The listing builds one solid part. Answer for the finished solid, in the listing's coordinates (mm). A direction names the side the tool comes from. Coordinates: 2 decimals unless noted, no trailing zeros. Loops run counter-clockwise (first coordinate to the right, second up) from the corner with the lowest first, then second, coordinate; pieces in that order, holes last. Notation, with made-up numbers: (15, 15) -> (38, 15) arc R32 cw to (38, 50) -> close; hole circle Ø4 at (18.25, 68). An arc over 180 degrees is marked (long way). Answer in a Markdown table with one row per item.
```python
from build123d import *

# Parameters (mm, degrees)
SKETCH1_R           = 50.8
SKETCH1_R_2         = 12.7
BOSS_EXTRUDE1_DEPTH = 3


with BuildPart() as part:
    # Sketch1 → Boss-Extrude1 (new body)
    with BuildSketch(Plane(origin=(0, 0, 0), x_dir=(1, 0, 0), z_dir=(0, 1, 0))):
        Circle(SKETCH1_R)
        Circle(SKETCH1_R_2, mode=Mode.SUBTRACT)
        with BuildLine():
            ThreePointArc((-33.25, 0), (-23.511300474, -23.511300474), (0, -33.25))
            ThreePointArc((0, -33.25), (1.5, -31.75), (0, -30.25))
            ThreePointArc((0, -30.25), (-21.389980131, -21.389980131), (-30.25, 0))
            ThreePointArc((-30.25, 0), (-31.75, 1.5), (-33.25, 0))
        make_face(mode=Mode.SUBTRACT)
        with BuildLine():
            ThreePointArc((-26.373662173, 5.295275591), (-19.021172414, -19.021172414), (5.295275591, -26.373662173))
            ThreePointArc((5.295275591, -26.373662173), (6.470650307, -24.607736275), (4.704724409, -23.432361559))
            ThreePointArc((4.704724409, -23.432361559), (-16.89985207, -16.89985207), (-23.432361559, 4.704724409))
            ThreePointArc((-23.432361559, 4.704724409), (-24.607736275, 6.470650307), (-26.373662173, 5.295275591))
        make_face(mode=Mode.SUBTRACT)
        with BuildLine():
            ThreePointArc((-20.55, 0), (-14.531044353, -14.531044353), (0, -20.55))
            ThreePointArc((0, -20.55), (1.5, -19.05), (0, -17.55))
            ThreePointArc((0, -17.55), (-12.40972401, -12.40972401), (-17.55, 0))
            ThreePointArc((-17.55, 0), (-19.05, 1.5), (-20.55, 0))
        make_face(mode=Mode.SUBTRACT)
    extrude(amount=BOSS_EXTRUDE1_DEPTH)


solid = part.part
```
Item 1: Find the intervals of material crossed by probe 1 along Z at (x, y) = (3, 0.6); probe 2 along X at (y, z) = (0.2, 21); probe 3 along Z at (x, y) = (-13.5, 0.2), in increasing order.
Findings below:
| item | result |
|---|---|
| probe 1 | z = -50.71 to -12.34, 12.34 to 23.71, 26.73 to 50.71 |
| probe 2 | x = -46.26 to -25.78, -21.77 to -16.81, -11.41 to 46.26 |
| probe 3 | z = -48.97 to 11.21, 15.49 to 19.72, 23.27 to 27.07, 30.39 to 48.97 |
Item 2: A tool of negligible diameter and unlimited length cuts with its end or side. For faces 5 (the face through (-23.77, 1.48, 23.25)), 6 (the face through (11, 0, -12)), from which of +Z, -Z, +X, -X, +Y, -Y can it reach the whole face along a straight path? Write none if from no direction.
Findings below:
| item | result |
|---|---|
| face 5 | +Y, -Y |
| face 6 | +Z, -Z, +X, -X, -Y |
Item 3: Determine the mould class of faces 1 (the face through (-11.012, 1.479, 49.592)), 2 (the face through (-19, 1.5, -1.5)), 3 (the face through (6.477, 1.479, 24.64)), 4 (the face through (11, 3, -12)) for opening direction Z: +Z half, -Z half, draft (parallel to the pull), parting line (faces both ways), or undercut.
Findings below:
| item | result |
|---|---|
| face 1 | parting line |
| face 2 | undercut |
| face 3 | undercut |
| face 4 | draft |
Item 4: A cutting plane is placed at D-D, the plane x = -5.5. Determine the outline of the cut face in (y, z).
Findings below:
| item | result |
|---|---|
| outline | (0, -50.5) -> (3, -50.5) -> (3, -11.45) -> (0, -11.45) -> close; (0, 11.45) -> (3, 11.45) -> (3, 16.67) -> (0, 16.67) -> close; (0, 19.8) -> (3, 19.8) -> (3, 23.26) -> (0, 23.26) -> close; (0, 26.33) -> (3, 26.33) -> (3, 29.75) -> (0, 29.75) -> close; (0, 32.79) -> (3, 32.79) -> (3, 50.5) -> (0, 50.5) -> close |
Item 5: A cutting plane is placed at A-A, the plane x = -19.05. Determine the outline of the cut face in (y, z).
Findings below:
| item | result |
|---|---|
| outline | (0, -47.09) -> (3, -47.09) -> (3, -1.5) -> (0, -1.5) -> close; (0, 7.71) -> (3, 7.71) -> (3, 14.43) -> (0, 14.43) -> close; (0, 18.99) -> (3, 18.99) -> (3, 23.5) -> (0, 23.5) -> close; (0, 27.25) -> (3, 27.25) -> (3, 47.09) -> (0, 47.09) -> close |
Item 6: A cutting plane is placed at B-B, the plane z = 6. Determine the outline of the cut face in (x, y).
Findings below:
| item | result |
|---|---|
| outline | (-50.44, 0) -> (-32.7, 0) -> (-32.7, 3) -> (-50.44, 3) -> close; (-29.65, 0) -> (-26.22, 0) -> (-26.22, 3) -> (-29.65, 3) -> close; (-23.13, 0) -> (-19.65, 0) -> (-19.65, 3) -> (-23.13, 3) -> close; (-16.49, 0) -> (-11.19, 0) -> (-11.19, 3) -> (-16.49, 3) -> close; (11.19, 0) -> (50.44, 0) -> (50.44, 3) -> (11.19, 3) -> close |
Item 7: A cutting plane is placed at C-C, the plane y = 1.25. Determine the outline of the cut face in (x, z), plus the area to 3 significant figures.
Findings below:
| item | result |
|---|---|
| outline | circle Ø101.6 at (0, 0); hole (-33.25, 0) arc R1.5 ccw to (-30.25, 0) arc R30.25 cw to (0, 30.25) arc R1.5 ccw to (0, 33.25) arc R33.25 ccw to start; hole (-26.37, -5.3) arc R1.5 ccw to (-23.43, -4.7) arc R23.9 cw to (4.7, 23.43) arc R1.5 ccw to (5.3, 26.37) arc R26.9 ccw to start; hole (-20.55, 0) arc R1.5 ccw to (-17.55, 0) arc R17.55 cw to (0, 17.55) arc R1.5 ccw to (0, 20.55) arc R20.55 ccw to start; hole circle Ø25.4 at (0, 0) |
| area | 7,190 mm2 |
